from build123d import *

# Parameters (mm, degrees)
F0_W      = 152.4
F0_H      = 127
F1_DEPTH  = 127
F2_W      = 101.6
F2_H      = 76.2
F3_DEPTH  = 88.9
F4_R      = 38.1
F5_DEPTH  = 25.4
F6_W      = 50.8
F6_H      = 50.8
F7_DEPTH  = 63.501
F8_SIZE   = 25.4
F9_R      = 17.6472220147
F10_DEPTH = 50.801


with BuildPart() as f1:
    # F0 (on Front) → F1 (new body)
    with BuildSketch(Plane.XZ):
        with Locations((9.334500879, 15.7128399368)):
            Rectangle(F0_W, F0_H)
    extrude(amount=F1_DEPTH)

    # F2 (on face) → F3 (cut)
    with BuildSketch(Plane.XZ.offset(127)):
        with Locations((34.734500879, 41.1128399368)):
            Rectangle(F2_W, F2_H)
    extrude(amount=-F3_DEPTH, mode=Mode.SUBTRACT)

    # F4
    f4_edges = [f1.edges().sort_by_distance(p)[0] for p in [
        (-41.465499, -127, 79.21284),
    ]]
    fillet(f4_edges, radius=F4_R)

    # F5 (add): a face of the model
    f5_faces = [f1.faces().sort_by_distance(p)[0] for p in [
        (34.734500879, -38.1, 41.1128399368),
    ]]
    extrude(f5_faces, amount=F5_DEPTH)

    # F6 (on face) → F7 (cut, through all)
    with BuildSketch(Plane.XZ.offset(63.5)):
        with Locations((9.334500879, 53.8128399368)):
            Rectangle(F6_W, F6_H)
    extrude(amount=-F7_DEPTH, mode=Mode.SUBTRACT)

    # F8
    f8_edges = [f1.edges().sort_by_distance(p)[0] for p in [
        (85.534501, -31.75, 79.21284),
    ]]
    chamfer(f8_edges, length=F8_SIZE)

    # F9 (on face) → F10 (cut, through all)
    with BuildSketch(Plane.XY.offset(3.0128399368)):
        with Locations((30.4336287081, -97.2528904676)):
            Circle(F9_R)
    extrude(amount=-F10_DEPTH, mode=Mode.SUBTRACT)


solid = f1.part
Read the model definition and answer for the solid it produces. Units are mm, in the model's axes. A direction names the side the tool comes from. Coordinates: 2 decimals unless noted, no trailing zeros. Order: outer loops, then holes, each group sorted by start corner. A loop starts at its lowest first (then second) coordinate and runs counter-clockwise, first axis right, second up. Notation, with made-up numbers: (-1, -6.5) - (8, -6.5) arc R26 cw to (8, 11.5) - close; hole circle Ø11 at (75, -6). An arc over 180 degrees is marked (long way). Use one line per item in the form item = value.
(1) Section C-C, the plane y = -12 is taken. Give the vertices of the cut face in (x, z), then the cut area to 3 significant figures.
Computed values:
outline = (-66.87, -47.79) - (85.53, -47.79) - (85.53, 53.81) - (60.13, 79.21) - (34.73, 79.21) - (34.73, 28.41) - (-16.07, 28.41) - (-16.07, 79.21) - (-66.87, 79.21) - close
area = 16,500 mm²
(2) Section A-A, the plane x = 22 is taken. Give the vertices of the cut face in (y, z), then the cut area to 3 significant figures.
Computed values:
outline = (-127, -47.79) - (-112.75, -47.79) - (-112.75, 3.01) - (-127, 3.01) - close; (-81.75, -47.79) - (0, -47.79) - (0, 28.41) - (-63.5, 28.41) - (-63.5, 3.01) - (-81.75, 3.01) - close
area = 6,490 mm²
(3) Section B-B, the plane z = 46.5 is taken. Give the vertices of the cut face in (x, y).
Computed values:
outline = (-66.87, -126.62) - (-16.07, -126.62) - (-16.07, 0) - (-66.87, 0) - close; (34.73, -63.5) - (85.53, -63.5) - (85.53, 0) - (34.73, 0) - close
(4) Straight lines are drawn through the part: L1, parallel to X at y = -15, z = 37; L2, parallel to X at y = -103, z = 32; L3, parallel to Z at x = 10.5, y = -117. For each, find the intervals that lie inside material, in ascending order.
Computed values:
L1 = -66.87 to -16.07, 34.73 to 85.53
L2 = -66.87 to -16.07
L3 = -47.79 to 3.01
(5) Section D-D, the plane x = 58 is taken. Give the vertices of the cut face in (y, z), then the cut area to 3 significant figures.
Computed values:
outline = (-127, -47.79) - (0, -47.79) - (0, 79.21) - (-63.5, 79.21) - (-63.5, 3.01) - (-127, 3.01) - close
area = 11,300 mm²
(6) For a pull along X with two mould halves and no side action, classify faces 1 (the face through (-16.065, -64, 41)), 2 (the face through (-66.865, -63, 15)), 3 (the face through (8, 0, 17)) as pulls with the +X half, pulls with the -X half, needs draft (parallel to the pull), parting line crosses it, or undercut.
Computed values:
face_1 = undercut
face_2 = pulls with the -X half
face_3 = needs draft
(7) Given pin 1 Ø1 at (x, z) = (-39, -5.5) entering from +Y; pin 2 Ø19 at (x, y) = (19.5, -105) entering from +Z; pin 3 Ø5 at (y, z) = (-110, 56.5) entering from +X; pin 4 Ø2 at (x, y) = (14, -51.5) entering from +Z, each flat-ended and moving along its own axis, determine where each tip first touches the part or whether it passes through.
Computed values:
pin_1 = 0
pin_2 = 3.01
pin_3 = -16.07
pin_4 = 28.41
(8) Which of the six approach directions +Z, -Z, +X, -X, +Y, -Y give full straight-line access (tool end or side, diameter ignored) to faces 4 (the face through (45, -82, 3.013)), 5 (the face through (9, -32, 28.413)), 6 (the face through (8, -63, -47.787))?
Computed values:
face_4 = +Z, +X, -Y
face_5 = +Z, +Y, -Y
face_6 = -Z, +X, -X, +Y, -Y
